The drawing under review shows one solid part. Ordinate dimensions are in mm from its lowest x, y, z. A direction names the side the tool comes from. Round coordinates to 2 decimals unless told otherwise and drop trailing zeros. Write each loop counter-clockwise with the first axis right and the second up, starting at its lowest first coordinate (ties: lowest second). Pieces come first, ordered by that corner, then holes. Notation, with made-up numbers: (-3, 52.25) -> (6, 52.25) arc R13 cw to (6, 68.25) -> close; hole circle Ø9 at (-33, -34.5). An arc over 180 degrees is marked (long way). Use CSV: the item, a comma, the result in double quotes. Start each with the question number.
1) Take a section at A-A, the plane x = 113.5. Give the boundary of the cut face in (y, z).
2) Take a section at B-B, the plane z = 215. Give the boundary of the cut face in (x, y), then the cut area to 3 significant figures.
3) For pin 1 Ø7.5 at (y, z) = (91.5, 268.5) entering from -X; pin 2 Ø5 at (x, z) = (200, 189) entering from -Y; pin 3 Ø7.5 at (y, z) = (90.5, 267.5) entering from +X, all flat-tipped, find the tip position at first contact; note any pin that passes through.
4) Take a section at C-C, the plane y = 111.5. Give the boundary of the cut face in (x, z).
5) Machinability: for the marked faces 1 and 2, which of the approach directions +Z, -Z, +X, -X, +Y, -Y give a long, thin tool a straight path to every point of the face, cutting with its end or side? Answer none if there is none.
6) Wall thickness on probe 1 along Y at (x, z) = (294, 23.5): over which ranges is the line inside the solid? List them lowest first. Write a range as [from, to].
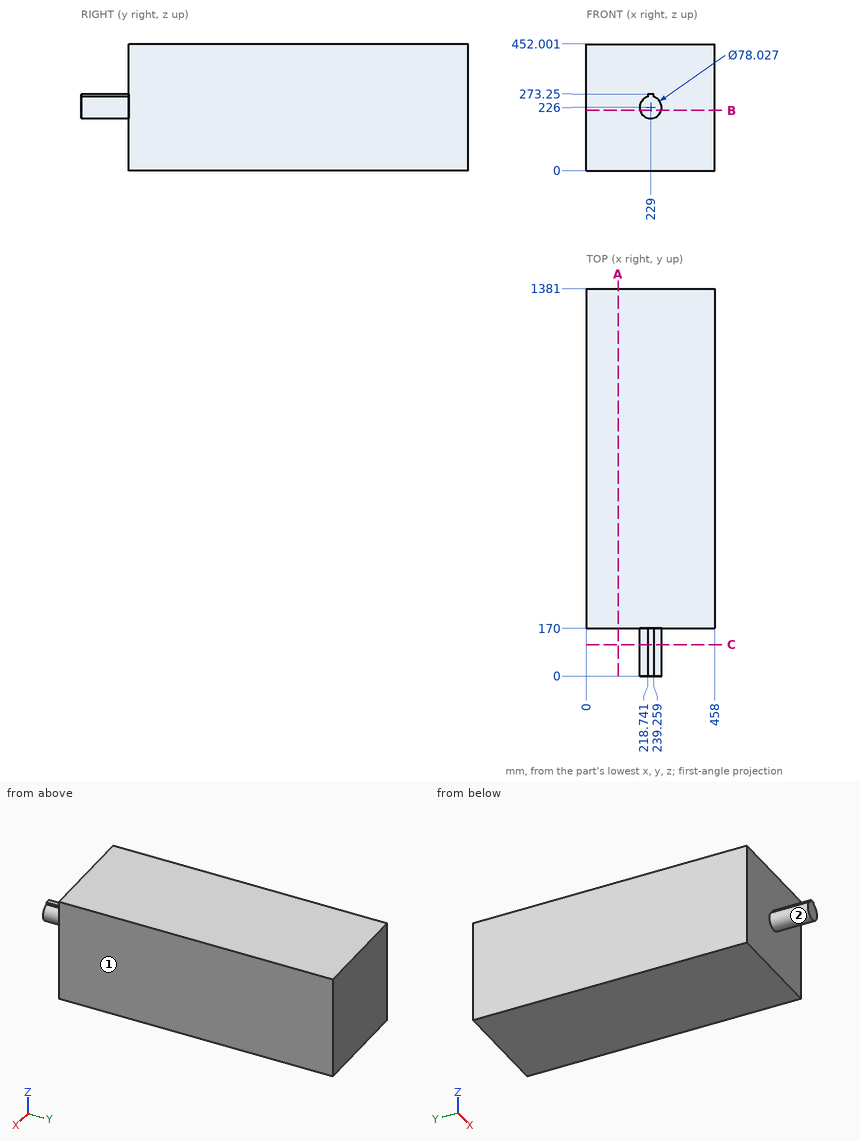
Values found:
1,outline,"(170, 0) -> (1381, 0) -> (1381, 452) -> (170, 452) -> close"
2,outline,"(0, 170) -> (191.57, 170) -> (191.57, 0) -> (266.43, 0) -> (266.43, 170) -> (458, 170) -> (458, 1381) -> (0, 1381) -> close"
2,area,"567,000 mm²"
3,pin 1,"x = 218.74"
3,pin 2,"y = 170"
3,pin 3,"x = 239.26"
4,outline,"(218.74, 263.64) arc R39.01 ccw (long way) to (239.26, 263.64) -> (239.26, 273.25) -> (218.74, 273.25) -> close"
5,face 1,"+Z, -Z, +X, +Y, -Y"
5,face 2,"-Y"
6,probe 1,"[170, 1381]"
